Input: part model. Units: mm. Frame: model coordinates. Face numbers are marked on the shaded views. Round coordinates to 2 decimals unless told otherwise and drop trailing zeros. Write each loop counter-clockwise with the first axis right and the second up, starting at its lowest first coordinate (ties: lowest second). Pieces come first, ordered by that corner, then holes. Notation, with made-up numbers: (85, 26.25) -> (108, 26.25) arc R23 ccw to (108, 53.25) -> close; hole circle Ø4 at (19, 78). An arc over 180 degrees is marked (long way). Write item = value, one per line.
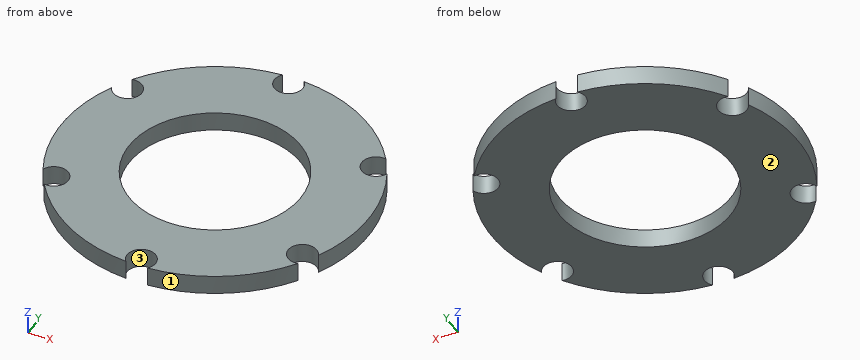
```python
from build123d import *

# Parameters (mm, degrees)
F0_R            = 25.4
F0_R_2          = 14.1605
F1_DEPTH        = 3.175
F2_R            = 2.3622
F3_DEPTH        = 3.176
F3_COPIES_COUNT = 6


# Not quite as in the source:
# - a pattern or mirror of a feature is missing from the dataset's text; its kind, count and spacing are read off the source's solid


with BuildPart() as f1:
    # F0 (on Top) → F1 (new body)
    with BuildSketch(Plane.XY):
        Circle(F0_R)
        Circle(F0_R_2, mode=Mode.SUBTRACT)
    extrude(amount=F1_DEPTH)

    # F2 (on face) → F3 (cut, through all)
    with BuildSketch(Plane.XY.offset(3.175)):
        with Locations((0, 23.8125)):
            Circle(F2_R)
    f3 = extrude(amount=-F3_DEPTH, mode=Mode.SUBTRACT)

    # F3_copies: F3 ×6 about axis
    f3_copies_axis = Axis((0, 0, 0), (0, 0, 1))
    for i in range(1, F3_COPIES_COUNT):
        add(f3.rotate(f3_copies_axis, i * 360 / F3_COPIES_COUNT), mode=Mode.SUBTRACT)


solid = f1.part
```
1) Line query: L1, parallel to X at y = 10.5, z = 1.8; L2, parallel to Y at x = 0, z = 2.1; L3, parallel to X at y = -12.5, z = 0.2. Output: solid intervals per line, ascending. Write a range as from..to.
Solutions:
L1 = -23.13..-22.52, -18.72..-9.5, 9.5..18.72, 22.52..23.13
L2 = -21.45..-14.16, 14.16..21.45
L3 = -18.34..-6.65, 6.65..18.34
2) Cut plane D-D (x = -16). Return the cut outline in (y, z) (3 decimals).
Solutions:
outline = (-19.727, 0) -> (19.727, 0) -> (19.727, 3.175) -> (-19.727, 3.175) -> close
3) Cut plane B-B (x = 0). Return the cut outline in (y, z) (1 decimal), and give its area (3 significant figures).
Solutions:
outline = (-21.5, 0) -> (-14.2, 0) -> (-14.2, 3.2) -> (-21.5, 3.2) -> close; (14.2, 0) -> (21.5, 0) -> (21.5, 3.2) -> (14.2, 3.2) -> close
area = 46.3 mm^2
4) Cut plane A-A (y = 0). Return the cut outline in (x, z) (1 decimal), and give its area (3 significant figures).
Solutions:
outline = (-25.4, 0) -> (-14.2, 0) -> (-14.2, 3.2) -> (-25.4, 3.2) -> close; (14.2, 0) -> (25.4, 0) -> (25.4, 3.2) -> (14.2, 3.2) -> close
area = 71.4 mm^2
5) Draft query along Y for the marked faces 1, 2 and 3. Return one class per face: +Y half, -Y half, draft (parallel to the pull), parting line (faces both ways), or undercut.
Solutions:
face_1 = -Y half
face_2 = draft
face_3 = undercut
6) Cut plane C-C (z = 2.4). Return the cut outline in (x, y), and give its area (3 significant figures).
Solutions:
outline = (-22.84, -11.1) arc R2.36 cw (long way) to (-21.04, -14.23) arc R25.4 ccw to (-1.81, -25.34) arc R2.36 cw (long way) to (1.81, -25.34) arc R25.4 ccw to (21.04, -14.23) arc R2.36 cw (long way) to (22.84, -11.1) arc R25.4 ccw to (22.84, 11.1) arc R2.36 cw (long way) to (21.04, 14.23) arc R25.4 ccw to (1.81, 25.34) arc R2.36 cw (long way) to (-1.81, 25.34) arc R25.4 ccw to (-21.04, 14.23) arc R2.36 cw (long way) to (-22.84, 11.1) arc R25.4 ccw to start; hole circle Ø28.32 at (0, 0)
area = 1,300 mm^2
